```python
from build123d import *
from OCP.BRepFilletAPI import BRepFilletAPI_MakeChamfer

# Parameters (mm, degrees)
SKETCH4_W                = 12.46
SKETCH4_H                = 17.25
BOSS_EXTRUDE3_DEPTH      = 6
BOSS_EXTRUDE6_DEPTH      = 7.3
BOSS_EXTRUDE6_DEPTH_BACK = 17.25
SKETCH8_R                = 12.546781182
SKETCH8_R_2              = 11.15
BOSS_EXTRUDE4_DEPTH      = 17.25
SKETCH6_R                = 2
CUT_EXTRUDE1_DEPTH       = 5
CHAMFER1_SIZE            = 0.5
CHAMFER1_SIZE_2          = 0.866025404
SKETCH10_W               = 12.46
SKETCH10_H               = 23.7
CUT_EXTRUDE3_DEPTH       = 17.25
CUT_EXTRUDE4_REACH       = 43.938
SKETCH11_W               = 5
SKETCH11_H               = 3
BOSS_EXTRUDE7_START      = -7.3
BOSS_EXTRUDE7_DEPTH      = 7.3
BOSS_EXTRUDE9_START      = 10
BOSS_EXTRUDE9_DEPTH      = 10
OFFSET_R_DEPTH           = 10


with BuildPart() as part:
    # Sketch4 → Boss-Extrude3 (new body)
    with BuildSketch(Plane.XY):
        with Locations((0, -1.35)):
            Rectangle(SKETCH4_W, SKETCH4_H)
    extrude(amount=BOSS_EXTRUDE3_DEPTH)



with BuildPart() as body_2:
    # Sketch8 → Boss-Extrude6 (new, two sides: drawn at the far end of the back side and taken through both)
    with BuildSketch(Plane(origin=(0, -9.975, 0), x_dir=(-1, 0, 0), z_dir=(0, -1, 0)).offset(-BOSS_EXTRUDE6_DEPTH_BACK)):
        with Locations(Location((0, -23.55, 0), (0, 0, 90))):
            Circle(SKETCH8_R)
        with Locations(Location((0, -23.55, 0), (0, 0, 90))):
            Circle(SKETCH8_R_2, mode=Mode.SUBTRACT)
    extrude(amount=BOSS_EXTRUDE6_DEPTH + BOSS_EXTRUDE6_DEPTH_BACK)


with BuildPart() as part_1:
    add(part.part)

    add(body_2.part)  # Boss-Extrude4 merges body 2
    # Sketch5 → Boss-Extrude4 (add)
    with BuildSketch(Plane(origin=(0, 7.275, 0), x_dir=(1, 0, 0), z_dir=(0, 1, 0))):
        with BuildLine():
            Line((12.546781182, -23.55), (12.546781182, 0))
            Line((12.546781182, 0), (6.23, 0))
            Line((6.23, 0), (6.23, -29.7))
            Line((6.23, -29.7), (-6.23, -29.7))
            Line((-6.23, -29.7), (-6.23, 0))
            Line((-6.23, 0), (-12.546781182, 0))
            Line((-12.546781182, 0), (-12.546781182, -23.55))
            ThreePointArc((-12.546781182, -23.55), (0, -36.096781182), (12.546781182, -23.55))
        make_face()
    extrude(amount=-BOSS_EXTRUDE4_DEPTH)

    # Sketch6 → Cut-Extrude1 (cut)
    with BuildSketch(Plane(origin=(0, 7.275, 0), x_dir=(1, 0, 0), z_dir=(0, 1, 0))):
        with Locations(Location((0, -3.5, 0), (0, 0, 270))):
            Circle(SKETCH6_R)
        with Locations(Location((0, -32.2, 0), (0, 0, 270))):
            Circle(SKETCH6_R)
    extrude(amount=-CUT_EXTRUDE1_DEPTH, mode=Mode.SUBTRACT)

    # Chamfer1
    chamfer1_edges_1 = [part_1.edges().sort_by_distance(p)[0] for p in [
        (0, 7.275, 1.5),
    ]]
    chamfer1_side_1 = [part_1.faces().sort_by_distance(p)[0] for p in [
        (0, 7.275, 1.49),
    ]]
    chamfer1_edges_2 = [part_1.edges().sort_by_distance(p)[0] for p in [
        (0, 7.275, 30.2),
    ]]
    chamfer1_side_2 = [part_1.faces().sort_by_distance(p)[0] for p in [
        (0, 7.275, 30.19),
    ]]
    chamfer1 = BRepFilletAPI_MakeChamfer(part_1.part.solid().wrapped)
    for e in chamfer1_edges_1:
        chamfer1.Add(CHAMFER1_SIZE - 0.0001, CHAMFER1_SIZE_2 - 0.0001, e.wrapped, chamfer1_side_1[0].wrapped)
    for e in chamfer1_edges_2:
        chamfer1.Add(CHAMFER1_SIZE - 0.0001, CHAMFER1_SIZE_2 - 0.0001, e.wrapped, chamfer1_side_2[0].wrapped)
    add(Compound.cast(chamfer1.Shape()), mode=Mode.REPLACE)  # a hair under: the kernel refuses the full size

    # Sketch10 → Cut-Extrude3 (cut)
    with BuildSketch(Plane(origin=(0, 7.275, 0), x_dir=(1, 0, 0), z_dir=(0, 1, 0))):
        with Locations((0, -17.85)):
            Rectangle(SKETCH10_W, SKETCH10_H)
    extrude(amount=-CUT_EXTRUDE3_DEPTH, mode=Mode.SUBTRACT)

    # Sketch11 → Cut-Extrude4 (cut, up to next)
    with BuildSketch(Plane.XY.offset(36.096781182), mode=Mode.PRIVATE) as cut_extrude4_sk1:
        with Locations((0, -8.475)):
            Rectangle(SKETCH11_W, SKETCH11_H)
    cut_extrude4_tool1 = extrude(cut_extrude4_sk1.sketch, amount=-CUT_EXTRUDE4_REACH, mode=Mode.PRIVATE) & part_1.part
    add(cut_extrude4_tool1.solids().sort_by_distance((0, -8.475, 36.096781))[0], mode=Mode.SUBTRACT)

    # Sketch13 → Boss-Extrude7 (add)
    with BuildSketch(Plane.XZ.offset(17.275).offset(BOSS_EXTRUDE7_START)):
        with BuildLine():
            Line((-12.546781182, 23.55), (-12.546781182, 0))
            Line((-12.546781182, 0), (12.546781182, 0))
            Line((12.546781182, 0), (12.546781182, 23.55))
            ThreePointArc((12.546781182, 23.55), (0, 11.003218818), (-12.546781182, 23.55))
        make_face()
    extrude(amount=BOSS_EXTRUDE7_DEPTH)

    # Sketch15 → Boss-Extrude9 (add)
    with BuildSketch(Plane(origin=(0, 7.275, 0), x_dir=(1, 0, 0), z_dir=(0, 1, 0)).offset(BOSS_EXTRUDE9_START)):
        with BuildLine():
            Line((-12.546781182, 0), (12.546781182, 0))
            Line((12.546781182, 0), (12.546781182, -23.55))
            ThreePointArc((12.546781182, -23.55), (0, -36.096781182), (-12.546781182, -23.55))
            Line((-12.546781182, -23.55), (-12.546781182, 0))
        make_face()
        with BuildLine():
            Line((-6.23, -0.8), (6.23, -0.8))
            Line((6.23, -0.8), (6.23, -33.5))
            ThreePointArc((6.23, -33.5), (5.937106781, -34.207106781), (5.23, -34.5))
            Line((5.23, -34.5), (-5.23, -34.5))
            ThreePointArc((-5.23, -34.5), (-5.937106781, -34.207106781), (-6.23, -33.5))
            Line((-6.23, -33.5), (-6.23, -0.8))
        make_face(mode=Mode.SUBTRACT)
    extrude(amount=-BOSS_EXTRUDE9_DEPTH)

    # Sketch1 → Offset R (add)
    with BuildSketch(Plane.XY):
        Polygon((0, -75), (74.307137052, 27.275), (-74.307137052, 27.275), align=None)
    extrude(amount=-OFFSET_R_DEPTH)


solid = part_1.part
```
The listing builds one solid part. Answer for the finished solid, in the listing's coordinates (mm). A direction names the side the tool comes from. Give positions to 0.01 mm unless a question says otherwise; leave off trailing zeros. Write each loop counter-clockwise with the first axis right and the second up, starting at its lowest first coordinate (ties: lowest second). Pieces come first, ordered by that corner, then holes. Notation, with made-up numbers: M 10.5,-2 L 62.5,-2 A32 cw 62.5,27 Z; hole C 31,46.5 d8. An arc over 180 degrees is marked long. Write each question's results on one line, items separated by ' | '.
Q1. A tool of negligible diameter and unlimited length cuts with its end or side. For faces 4 (the flat face through (12.547, 0, 12)), 5 (the flat face through (-2.5, -8, 33)), 6 (the flat face through (-1.5, 7.275, 29.9)), from which of +Z, -Z, +X, -X, +Y, -Y can it reach the whole face along a straight path? Write none if from no direction.
Output values:
face 4: +Z, +X, +Y, -Y | face 5: +Z | face 6: +Y
Q2. Flat-ended cylindrical pins translate along their axes: P1, Ø1.5, axis at y = -9, z = 31.5, coming from the +X side; P2, Ø13.5, axis at x = 2.5, y = -4.5, coming from the +Z side; P3, Ø10, axis at x = -15, z = 15.5, coming from the -Y side (3 decimals); P4, Ø22, axis at y = 9.5, z = 18.5, coming from the +X side. Find the tip coordinate at first contact, or state that the pin passes through.
Output values:
P1: x = 10.28 | P2: z = 36.1 | P3: y = -17.275 | P4: x = 12.55
Q3. Consider L1, parallel to Z at x = 0, y = -14; L2, parallel to X at y = 3.7, z = 3.5; L3, parallel to Z at x = -29, y = -33. Determine where each line is inside the solid, lowest interval first. Write a range as from..to.
Output values:
L1: -10..12.4, 34.7..36.1 | L2: -12.55..-2, 2..12.55 | L3: -10..0
Q4. Section A-A, the plane z = 3.5 is taken. Write down the section's boundary in (x, y) (3 decimals), then the cut area to 3 significant figures.
Output values:
outline: M -12.547,-17.275 L 12.547,-17.275 L 12.547,17.275 L 6.23,17.275 L 6.23,7.275 L 2.5,7.275 L 2,6.409 L 2,2.275 L -2,2.275 L -2,6.409 L -2.5,7.275 L -6.23,7.275 L -6.23,17.275 L -12.547,17.275 Z | area: 722 mm2
Q5. For a pull along Z with two mould halves and no side action, classify faces 1 (the flat face through (-1, -12, -10)), 2 (the flat face through (8, -9.975, 24)), 3 (the flat face through (-37.67, -23.15, -4.93)) as released by +Z, released by -Z, zero draft, split by the parting line, or undercut.
Output values:
face 1: released by -Z | face 2: undercut | face 3: zero draft
Q6. Section C-C, the plane x = -40 is taken. Write down the section's boundary in (y, z) (3 decimals).
Output values:
outline: M -19.945,-10 L 27.275,-10 L 27.275,0 L -19.945,0 Z
Q7. Section B-B, the plane y = -64 is taken. Write down the section's boundary in (x, z).
Output values:
outline: M -7.99,-10 L 7.99,-10 L 7.99,0 L -7.99,0 Z
